from build123d import *

# Parameters (mm, degrees)
SKETCH1_R           = 1.5
BOSS_EXTRUDE1_DEPTH = 1.61
FILLET1_R           = 3


with BuildPart() as part:
    # Sketch1 → Boss-Extrude1 (new body, symmetric)
    with BuildSketch(Plane.XY):
        Polygon((-7, 12.5), (-15, 12.5), (-15, 22.5), (15, 22.5), (15, 12.5), (7, 12.5), (7, -12.5), (-7, -12.5), align=None)
        with Locations((-7.5, 15.5)):
            Circle(SKETCH1_R, mode=Mode.SUBTRACT)
        with Locations((0, 15.5)):
            Circle(SKETCH1_R, mode=Mode.SUBTRACT)
        with Locations((7.5, 15.5)):
            Circle(SKETCH1_R, mode=Mode.SUBTRACT)
        with Locations((0, -4.5)):
            Circle(SKETCH1_R, mode=Mode.SUBTRACT)
    extrude(amount=BOSS_EXTRUDE1_DEPTH, both=True)

    # Fillet1
    fillet1_edges = [part.edges().sort_by_distance(p)[0] for p in [
        (7, 12.5, 0),
        (7, -12.5, 0),
        (-7, -12.5, 0),
        (-7, 12.5, 0),
        (-15, 12.5, 0),
        (-15, 22.5, 0),
        (15, 22.5, 0),
        (15, 12.5, 0),
    ]]
    fillet(fillet1_edges, radius=FILLET1_R)


solid = part.part
Input: part model. Units: mm. Frame: model coordinates. A direction names the side the tool comes from. Coordinates: 2 decimals unless noted, no trailing zeros. Loops run counter-clockwise (first coordinate to the right, second up) from the corner with the lowest first, then second, coordinate; pieces in that order, holes last. Notation, with made-up numbers: (-26.75, 10) -> (19.25, 10) arc R15 cw to (19.25, 34) -> close; hole circle Ø8 at (-34.5, 14). An arc over 180 degrees is marked (long way). Write each question's results on one line, items separated by ' | '. Start each with the question number.
Q1. Ray query, line 1 (Y direction, x = 0, z = 0.05); line 2 (Y direction, x = 7.5, z = 0.6); line 3 (X direction, y = 5.5, z = 0.8). Return the intervals inside material, ascending. Write a range as from..to.
Q2. Section A-A, the plane y = -4.5. Return the cut outline in (x, z), plus the area to 3 significant figures.
Q3. Section B-B, the plane z = -0.6. Return the cut outline in (x, y), plus the area to 3 significant figures.
Q4. Pull-direction query (Y, two-part tool) for faces 4 (the flat face through (-11, 12.5, 0)), 5 (the cylindrical face through (14.14, 21.6, -0.02)), 6 (the cylindrical face through (-1.11, 16.51, -0.02)), 7 (the flat face through (15, 18, 0)); classes: released by +Y, released by -Y, zero draft, split by the parting line, or undercut.
Q5. Reachability of faces 1 (the flat face through (7, 0, 0)), 2 (the flat face through (-7, 0, 0)), 3 (the flat face through (0, 22.5, 0)) from +Z, -Z, +X, -X, +Y, -Y: full face, straight path, thin tool, end or side. Return the list, or none.
Q6. Pin query (flat end, axial travel): pin 1 (0.6 mm diameter, centred on x = 11.5, z = -0.5, fed in from -Y); pin 2 (1.6 mm diameter, centred on y = -3.5, z = -0.5, fed in from +X); pin 3 (2.5 mm diameter, centred on x = -7.5, y = 15.5, fed in from +Z); pin 4 (1.6 mm diameter, centred on y = 0.5, z = -0.5, fed in from -X). Return the tip coordinate at first contact, or that it passes through.
Q7. Section D-D, the plane x = 7.5. Return the cut outline in (y, z).
Q8. Section C-C, the plane x = 0. Return the cut outline in (y, z).
Found:
1) line 1: -12.5..-6, -3..14, 17..22.5 | line 2: 11.16..14, 17..22.5 | line 3: -7..7
2) outline: (-7, -1.61) -> (-1.5, -1.61) -> (-1.5, 1.61) -> (-7, 1.61) -> close; (1.5, -1.61) -> (7, -1.61) -> (7, 1.61) -> (1.5, 1.61) -> close | area: 35.4 mm2
3) outline: (-15, 15.5) arc R3 ccw to (-12, 12.5) -> (-10, 12.5) arc R3 cw to (-7, 9.5) -> (-7, -9.5) arc R3 ccw to (-4, -12.5) -> (4, -12.5) arc R3 ccw to (7, -9.5) -> (7, 9.5) arc R3 cw to (10, 12.5) -> (12, 12.5) arc R3 ccw to (15, 15.5) -> (15, 19.5) arc R3 ccw to (12, 22.5) -> (-12, 22.5) arc R3 ccw to (-15, 19.5) -> close; hole circle Ø3 at (-7.5, 15.5); hole circle Ø3 at (0, -4.5); hole circle Ø3 at (0, 15.5); hole circle Ø3 at (7.5, 15.5) | area: 614 mm2
4) face 4: released by -Y | face 5: released by +Y | face 6: undercut | face 7: zero draft
5) face 1: +Z, -Z, +X, -Y | face 2: +Z, -Z, -X, -Y | face 3: +Z, -Z, +X, -X, +Y
6) pin 1: y = 12.5 | pin 2: x = 7 | pin 3: through | pin 4: x = -7
7) outline: (11.16, -1.61) -> (14, -1.61) -> (14, 1.61) -> (11.16, 1.61) -> close; (17, -1.61) -> (22.5, -1.61) -> (22.5, 1.61) -> (17, 1.61) -> close
8) outline: (-12.5, -1.61) -> (-6, -1.61) -> (-6, 1.61) -> (-12.5, 1.61) -> close; (-3, -1.61) -> (14, -1.61) -> (14, 1.61) -> (-3, 1.61) -> close; (17, -1.61) -> (22.5, -1.61) -> (22.5, 1.61) -> (17, 1.61) -> close
